from build123d import *

# Parameters (mm, degrees)
F1_DEPTH = 2.54
F3_DEPTH = 25.4
F4_R     = 1.55
F4_R_2   = 1.884603
F5_DEPTH = 25.4


with BuildPart() as f1:
    # F0 (on Top) → F1 (new body)
    with BuildSketch(Plane.XY):
        Polygon((25.3638, 76.552555), (-53.614557, 60.241973), (-78.978357, -16.310582), (-25.3638, -76.552555), (53.614557, -60.241973), (78.978357, 16.310582), align=None)
    extrude(amount=F1_DEPTH)

    # F2 (on face) → F3 (cut)
    with BuildSketch(Plane.XY.offset(2.54)):
        with BuildLine():
            ThreePointArc((24.21445, 68.483899), (23.925977, 69.376115), (23.169766, 69.930562))
            ThreePointArc((23.169766, 69.930562), (21.454923, 67.591684), (24.21445, 68.483899))
        make_face()
        with BuildLine():
            ThreePointArc((-46.439572, 53.892456), (-47.339682, 55.282901), (-48.97676, 55.030887))
            ThreePointArc((-48.97676, 55.030887), (-48.587461, 52.502011), (-46.439572, 53.892456))
        make_face()
        with BuildLine():
            ThreePointArc((-21.16645, -68.483899), (-23.582666, -67.248373), (-23.169766, -69.930562))
            ThreePointArc((-23.169766, -69.930562), (-21.798234, -69.719426), (-21.16645, -68.483899))
        make_face()
        with BuildLine():
            ThreePointArc((49.487572, -53.892456), (46.573126, -53.268566), (48.97676, -55.030887))
            ThreePointArc((48.97676, -55.030887), (49.354017, -54.516346), (49.487572, -53.892456))
        make_face()
    extrude(amount=-F3_DEPTH, mode=Mode.SUBTRACT)

    # F4 (on face) → F5 (cut)
    with BuildSketch(Plane.XY.offset(2.54)):
        with Locations((37.449616, -47.753262)):
            Circle(F4_R)
        with Locations((-12.550384, -64.205859)):
            Circle(F4_R)
        with Locations((22.179618, 26.186424)):
            Circle(F4_R_2)
        with Locations((-24.820382, 17.501104)):
            Circle(F4_R)
    extrude(amount=-F5_DEPTH, mode=Mode.SUBTRACT)


solid = f1.part
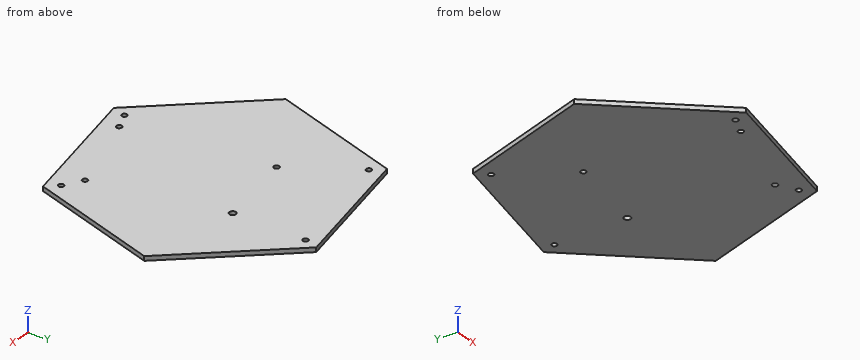
Source: CAD feature listing. Evaluate the final solid. Frame: model axes, mm. Coordinates: 2 decimals unless noted, no trailing zeros. Loops run counter-clockwise (first coordinate to the right, second up) from the corner with the lowest first, then second, coordinate; pieces in that order, holes last. Notation, with made-up numbers: M 13,-35.5 L 44,-35.5 A15 ccw 44,-9.5 Z; hole C -28.5,71.25 d11. An arc over 180 degrees is marked long. Answer in a Markdown table with one row per item.
Q1. Section B-B on x = -66.5. Return the cut outline in (y, z), plus the area to 3 significant figures.
Answers below:
| item | result |
|---|---|
| outline | M -30.33,0 L 21.35,0 L 21.35,2.54 L -30.33,2.54 Z |
| area | 131 mm^2 |
Q2. Ray query, probe 1 along Y at (x, z) = (47.5, 2.3); probe 2 along Y at (x, z) = (-23, 1.05); probe 3 along Y at (x, z) = (12.5, 0.6). Return the intervals inside material, ascending. Write a range as from..to.
Answers below:
| item | result |
|---|---|
| probe 1 | y = -61.5..-55.34, -52.44..51.68 |
| probe 2 | y = -76.06..-69.98, -66.99..66.56 |
| probe 3 | y = -68.73..73.9 |
Q3. First-contact query: pin 1 (1 mm diameter, centred on y = 43.5, z = 2, fed in from +X). Flat tip, straight axial feed; report the tip coordinate or a pass-through.
Answers below:
| item | result |
|---|---|
| pin 1 | stops at x = 55.23 |
Q4. Section A-A on z = 1.5. State how many separate pieces and enclosed holes the cut face has, plus the area to 3 significant figures.
Answers below:
| item | result |
|---|---|
| separate pieces | 1 |
| enclosed holes | 8 |
| area | 16,800 mm^2 |
Q5. Section C-C on y = -25.5. Return the cut outline in (x, z).
Answers below:
| item | result |
|---|---|
| outline | M -70.8,0 L 65.13,0 L 65.13,2.54 L -70.8,2.54 Z |
